Drawing for the job (mm, zero at the part's lowest x, y, z). Coordinates: 2 decimals unless noted, no trailing zeros. Write each loop counter-clockwise with the first axis right and the second up, starting at its lowest first coordinate (ties: lowest second). Pieces come first, ordered by that corner, then holes. Notation, with made-up numbers: (42, 36.5) -> (53, 36.5) arc R17 ccw to (53, 48.5) -> close; hole circle Ø9 at (7, 13.5). An arc over 180 degrees is marked (long way). Write each question's results on one line, items separated by ' | '. Start each with the question number.
Q1. Drop flat-ended pins along their axis: pin 1 Ø10 at (y, z) = (15, 28.5) entering from +X; pin 2 Ø1 at (y, z) = (17, 31) entering from +X; pin 3 Ø10 at (y, z) = (20, 11) entering from +X. Give the stop position or say it passes through.
Q2. Saw through at B-B on y = 25. Give the cut face in (x, z).
Q3. Two-plate mould, pull along X, no slides. Class the marked faces 1, 2 and 3: released by +X, released by -X, zero draft, split by the parting line, or undercut.
Q4. Saw through at A-A on x = 35. Give the cut face in (y, z).
Q5. Saw through at D-D on x = 53. Give the cut face in (y, z).
Q6. Drill centre lines: line 1 (Y direction, x = 35, z = 25); line 2 (X direction, y = 23, z = 20); line 3 (Y direction, x = 48.5, z = 5). Where is each one in solid material? Low to high.
Q7. Saw through at C-C on z = 27. Give the cut face in (x, y), and give its area (3 significant figures).
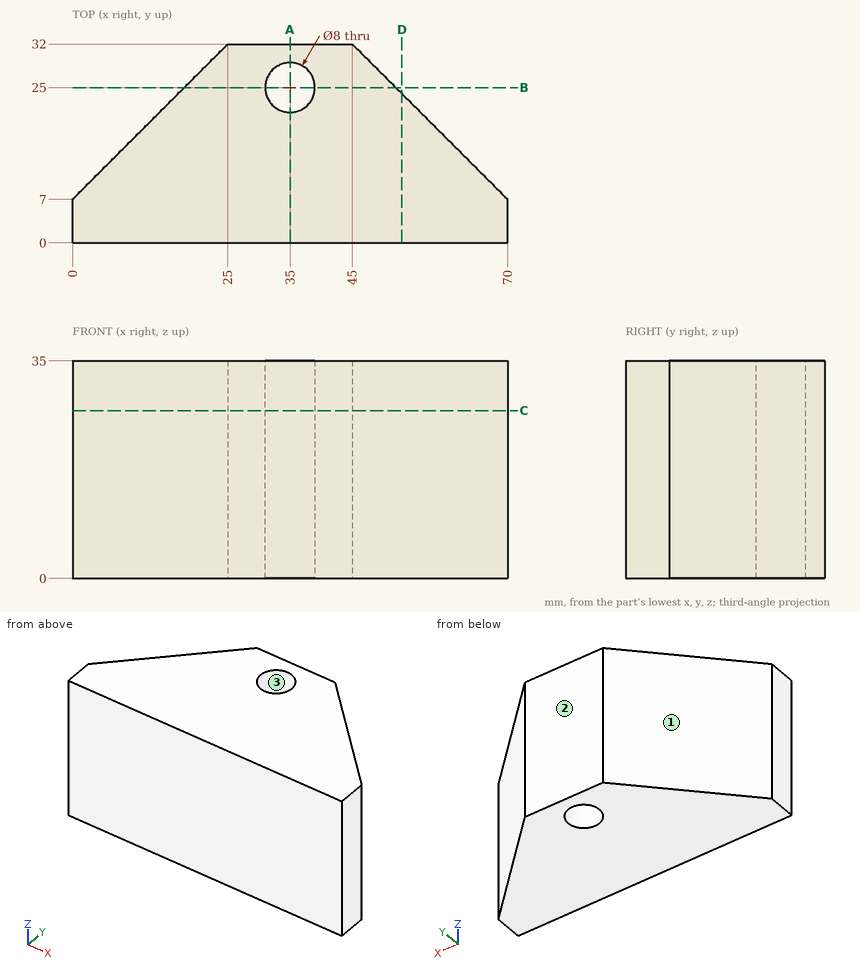
Returned:
1) pin 1: stops at x = 67 | pin 2: stops at x = 60.5 | pin 3: stops at x = 62
2) outline: (18, 0) -> (31, 0) -> (31, 35) -> (18, 35) -> close; (39, 0) -> (52, 0) -> (52, 35) -> (39, 35) -> close
3) face 1: released by -X | face 2: zero draft | face 3: undercut
4) outline: (0, 0) -> (21, 0) -> (21, 35) -> (0, 35) -> close; (29, 0) -> (32, 0) -> (32, 35) -> (29, 35) -> close
5) outline: (0, 0) -> (24, 0) -> (24, 35) -> (0, 35) -> close
6) line 1: y = 0 to 21, 29 to 32 | line 2: x = 16 to 31.54, 38.46 to 54 | line 3: y = 0 to 28.5
7) outline: (0, 0) -> (70, 0) -> (70, 7) -> (45, 32) -> (25, 32) -> (0, 7) -> close; hole circle Ø8 at (35, 25) | area: 1,560 mm2
